Check sheet for the modelled part. Datum: model origin and axes. Units: mm. A direction names the side the tool comes from. Give positions to 0.01 mm unless a question says otherwise; leave off trailing zeros. Write each loop counter-clockwise with the first axis right and the second up, starting at its lowest first coordinate (ties: lowest second). Pieces come first, ordered by that corner, then holes. Notation, with made-up numbers: (89, 19.25) -> (128, 19.25) arc R16 ccw to (128, 42.25) -> close; hole circle Ø6 at (85.5, 40.25). An arc over 180 degrees is marked (long way). Use a Markdown table: item, result. Add a question column.
1. Cross-section at C-C (x = 21). Enter the section's corners in (y, z), then the cut area to 3 significant figures.
2. Release check for a two-part mould opening along Y. For faces 5 (the flat face through (2, 5, -30)), 6 (the flat face through (5, 11, -16)), 7 (the flat face through (18.25, 11, -2)) record: released by +Y, released by -Y, zero draft, split by the parting line, or undercut.
3. Cross-section at B-B (y = 9.5). Enter the section's corners in (x, z).
4. Cross-section at A-A (x = 16). Enter the section's corners in (y, z).
5. Set-up check for faces 1 (the flat face through (14, 11, -28.05)), 2 (the flat face through (23.25, 11, -29)), 3 (the cylindrical face through (20.78, 11.99, -2.64)), 4 (the flat face through (2, 5, -2)): record each of +Z, -Z, +X, -X, +Y, -Y from which the full face is reachable in a straight line by a thin tool's end or side.
6. Gauge pin test, flat ends, axial feed: P1, Ø3.5, axis at x = 13.5, y = 10, coming from the +Z side; P2, Ø4, axis at x = 12, z = -8.5, coming from the +Y side; P3, Ø5, axis at y = 8.5, z = -6, coming from the +X side; P4, Ø1.6, axis at y = 11.15, z = -30.2, coming from the +X side. Record the tip position at first contact, or that the pin passes through.
7. Cross-section at D-D (z = -20). Enter the section's corners in (x, y).
8. Scan lines: probe 1 along Z at (x, y) = (8, 15.25); probe 2 along X at (y, z) = (3.75, -2.5); probe 3 along Z at (x, y) = (3, 2). Record each from-to range of solid material in increasing order. Write a range as [from, to].
from build123d import *

# Parameters (mm, degrees)
SKETCH4_W           = 35
SKETCH4_H           = 32.3
BOSS_EXTRUDE3_DEPTH = 5
SKETCH6_W           = 5
SKETCH6_H           = 32.3
BOSS_EXTRUDE5_DEPTH = 12.2
SKETCH8_W           = 18.25
SKETCH8_H           = 4.25
BOSS_EXTRUDE6_DEPTH = 12.2
SKETCH10_R          = 1
CUT_EXTRUDE1_DEPTH  = 5
SKETCH11_R          = 1
CUT_EXTRUDE2_DEPTH  = 5
SKETCH12_R          = 1
CUT_EXTRUDE3_DEPTH  = 5
FILLET2_R           = 2


with BuildPart() as part:
    # Sketch4 → Boss-Extrude3 (new body)
    with BuildSketch(Plane(origin=(0, 0, 0), x_dir=(1, 0, 0), z_dir=(0, 1, 0))):
        with Locations((17.5, 16.15)):
            Rectangle(SKETCH4_W, SKETCH4_H)
    extrude(amount=BOSS_EXTRUDE3_DEPTH)

    # Sketch6 → Boss-Extrude5 (add)
    with BuildSketch(Plane(origin=(0, 5, 0), x_dir=(1, 0, 0), z_dir=(0, 1, 0))):
        with Locations((2.5, 16.15)):
            Rectangle(SKETCH6_W, SKETCH6_H)
    extrude(amount=BOSS_EXTRUDE5_DEPTH)

    # Sketch8 → Boss-Extrude6 (add)
    with BuildSketch(Plane(origin=(0, 5, 0), x_dir=(1, 0, 0), z_dir=(0, 1, 0))):
        with Locations((14.125, 2.125)):
            Rectangle(SKETCH8_W, SKETCH8_H)
        with Locations((14.125, 30.175)):
            Rectangle(SKETCH8_W, SKETCH8_H)
    extrude(amount=BOSS_EXTRUDE6_DEPTH)

    # Sketch10 → Cut-Extrude1 (cut)
    with BuildSketch(Plane(origin=(23.25, 0, 0), x_dir=(0, 0, -1), z_dir=(1, 0, 0))):
        with Locations((2.1, 11.15)):
            Circle(SKETCH10_R)
        with Locations((30.2, 11.15)):
            Circle(SKETCH10_R)
    extrude(amount=-CUT_EXTRUDE1_DEPTH, mode=Mode.SUBTRACT)

    # Sketch11 → Cut-Extrude2 (cut)
    with BuildSketch(Plane(origin=(0, 5, 0), x_dir=(1, 0, 0), z_dir=(0, 1, 0))):
        with BuildLine():
            ThreePointArc((28.65708215, 30.175), (27.65708215, 31.175), (26.65708215, 30.175))
            Line((26.65708215, 30.175), (28.65708215, 30.175))
        make_face()
        with BuildLine():
            Line((28.65708215, 30.175), (26.65708215, 30.175))
            ThreePointArc((26.65708215, 30.175), (27.65708215, 29.175), (28.65708215, 30.175))
        make_face()
        with BuildLine():
            ThreePointArc((33.028108072, 30.175), (32.028108072, 31.175), (31.028108072, 30.175))
            Line((31.028108072, 30.175), (33.028108072, 30.175))
        make_face()
        with BuildLine():
            Line((33.028108072, 30.175), (31.028108072, 30.175))
            ThreePointArc((31.028108072, 30.175), (32.028108072, 29.175), (33.028108072, 30.175))
        make_face()
        with Locations((27.65708215, 2.125)):
            Circle(SKETCH11_R)
        with Locations((32.028108072, 2.125)):
            Circle(SKETCH11_R)
    extrude(amount=-CUT_EXTRUDE2_DEPTH, mode=Mode.SUBTRACT)

    # Sketch12 → Cut-Extrude3 (cut)
    with BuildSketch(Plane.XZ):
        with Locations((2.322349093, -2.125)):
            Circle(SKETCH12_R)
        with Locations((2.322349093, -30.175)):
            Circle(SKETCH12_R)
    extrude(amount=-CUT_EXTRUDE3_DEPTH, mode=Mode.SUBTRACT)

    # Fillet2
    fillet2_edges = [part.edges().sort_by_distance(p)[0] for p in [
        (35, 2.5, -32.3),
        (35, 2.5, 0),
    ]]
    fillet(fillet2_edges, radius=FILLET2_R)


solid = part.part
Worked answers:
| question | item | result |
|---|---|---|
| 1 | outline | (0, -32.3) -> (17.2, -32.3) -> (17.2, -28.05) -> (5, -28.05) -> (5, -4.25) -> (17.2, -4.25) -> (17.2, 0) -> (0, 0) -> close; hole circle Ø2 at (11.15, -30.2); hole circle Ø2 at (11.15, -2.1) |
| 1 | area | 259 mm² |
| 2 | face 5 | released by -Y |
| 2 | face 6 | zero draft |
| 2 | face 7 | undercut |
| 3 | outline | (0, -32.3) -> (23.25, -32.3) -> (23.25, -28.05) -> (5, -28.05) -> (5, -4.25) -> (23.25, -4.25) -> (23.25, 0) -> (0, 0) -> close |
| 4 | outline | (0, -32.3) -> (17.2, -32.3) -> (17.2, -28.05) -> (5, -28.05) -> (5, -4.25) -> (17.2, -4.25) -> (17.2, 0) -> (0, 0) -> close |
| 5 | face 1 | +X, +Y |
| 5 | face 2 | +Z, -Z, +X, +Y |
| 5 | face 3 | +X |
| 5 | face 4 | -Y |
| 6 | P1 | stops at z = 0 |
| 6 | P2 | stops at y = 5 |
| 6 | P3 | stops at x = 23.25 |
| 6 | P4 | stops at x = 18.25 |
| 7 | outline | (0, 0) -> (35, 0) -> (35, 5) -> (5, 5) -> (5, 17.2) -> (0, 17.2) -> close |
| 8 | probe 1 | z = [-32.3, -28.05], [-4.25, 0] |
| 8 | probe 2 | x = [0, 1.4], [3.25, 26.73], [28.58, 31.1], [32.96, 35] |
| 8 | probe 3 | z = [-32.3, -30.91], [-29.44, -2.86], [-1.39, 0] |
